Can you work these out from the model? Positions are in its coordinate system, mm. Face numbers are marked on the shaded views. A direction names the side the tool comes from. Round coordinates to 2 decimals unless told otherwise and drop trailing zeros. Order: outer loops, then holes, each group sorted by start corner. A loop starts at its lowest first (then second) coordinate and runs counter-clockwise, first axis right, second up.
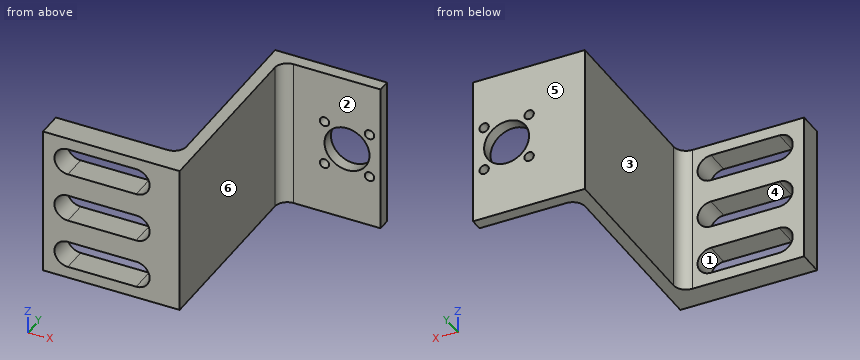
from build123d import *

# Parameters (mm, degrees)
BOSS_EXTRUDE1_DEPTH  = 19.05
FILLET1_R            = 3.175
SKETCH2_R            = 5.75
CUT_EXTRUDE1_DEPTH   = 4.175
M2_CLEARANCE_HOLE1_D = 2.4
CUT_EXTRUDE2_DEPTH   = 7.35
LPATTERN1_COUNT      = 2
LPATTERN1_PITCH      = 12.7
LPATTERN1_COL_COUNT  = 2
LPATTERN1_COL_PITCH  = 12.7


with BuildPart() as part:
    # Sketch1 → Boss-Extrude1 (new body, symmetric)
    with BuildSketch(Plane.XY):
        Polygon((-34.925, 0), (0, 0), (0, 50.2412), (25.4, 50.2412), (25.4, 53.4162), (-3.175, 53.4162), (-3.175, 6.35), (-34.925, 6.35), align=None)
    extrude(amount=BOSS_EXTRUDE1_DEPTH, both=True)

    # Fillet1
    fillet1_edges = [part.edges().sort_by_distance(p)[0] for p in [
        (-3.175, 6.35, 0),
        (0, 50.2412, 0),
    ]]
    fillet(fillet1_edges, radius=FILLET1_R)

    # Sketch2 → Cut-Extrude1 (cut, through all)
    with BuildSketch(Plane(origin=(16.8125, 50.2412, 0), x_dir=(1, 0, 0), z_dir=(0, -1, 0))):
        Circle(SKETCH2_R)
    extrude(amount=-CUT_EXTRUDE1_DEPTH, mode=Mode.SUBTRACT)

    # M2 Clearance Hole1 (through all)
    with Locations(Plane(origin=(16.8125, 50.2412, 0), x_dir=(-1, 0, 0), z_dir=(0, -1, 0))):
        with Locations((-5.75, -5.75), (-5.75, 5.75), (5.75, 5.75), (5.75, -5.75)):
            Hole(M2_CLEARANCE_HOLE1_D / 2)

    # Sketch5 → Cut-Extrude2 (cut, through all)
    with BuildSketch(Plane(origin=(0, 6.35, 0), x_dir=(1, 0, 0), z_dir=(0, 1, 0))):
        with BuildLine():
            Line((-28.575, 3.429), (-11.1125, 3.429))
            ThreePointArc((-11.1125, 3.429), (-7.6835, 0), (-11.1125, -3.429))
            Line((-11.1125, -3.429), (-28.575, -3.429))
            ThreePointArc((-28.575, -3.429), (-32.004, 0), (-28.575, 3.429))
        make_face()
    cut_extrude2 = extrude(amount=-CUT_EXTRUDE2_DEPTH, mode=Mode.SUBTRACT)

    # LPattern1: Cut-Extrude2 ×2
    with Locations(*[(0, 0, i * LPATTERN1_PITCH) for i in range(1, LPATTERN1_COUNT)]):
        add(cut_extrude2, mode=Mode.SUBTRACT)

    # LPattern1 col: Cut-Extrude2 ×2
    with Locations(*[(0, 0, -i * LPATTERN1_COL_PITCH) for i in range(1, LPATTERN1_COL_COUNT)]):
        add(cut_extrude2, mode=Mode.SUBTRACT)


solid = part.part
(1) I want a section at B-B, the plane z = 1. List the corners of the cut face in (x, y) for me (3 decimals).
(2) On a 3-axis mill with a long thin cutter (end or side, diameter ignored), from which of +Z, -Z, +X, -X, +Y, -Y can I reach the whole of each face in a straight line? I mean the marked faces 1, 2 and 3. Say none if no direction works.
(3) Please list where these lines run through material, in increasing order: probe 1 along X at (y, z) = (24, 8) (3 decimals); probe 2 along Y at (x, z) = (-8.5, 15); probe 3 along X at (y, z) = (51.5, 1) (3 decimals).
(4) If we mould it in two halves opening along X, with no side actions, what happens to the marked faces 4, 5 and 6? For each: pulls with the +X half, pulls with the -X half, needs draft (parallel to the pull), parting line crosses it, or undercut.
(5) I'm going to push flat-ended pins straight in: pin 1 Ø4 at (x, z) = (-6, 12.5) entering from +Y; pin 2 Ø12 at (y, z) = (25.5, 10.5) entering from +X; pin 3 Ø1.4 at (x, z) = (22.56, 5.75) entering from -Y; pin 4 Ø11 at (x, z) = (12.5, -7) entering from -Y. Where does each tip first touch, or does it pass through?
(6) I want a section at D-D, the plane x = 9. List the corners of the cut face in (y, z) for me.
(7) I want a section at C-C, the plane y = 16. List the corners of the cut face in (x, z) for me (3 decimals).
Ans:
1. outline: (-34.925, 0) - (-31.855, 0) - (-31.855, 6.35) - (-34.925, 6.35) - close; (-7.833, 0) - (0, 0) - (0, 47.066) arc R3.175 cw to (3.175, 50.241) - (11.15, 50.241) - (11.15, 53.416) - (-3.175, 53.416) - (-3.175, 9.525) arc R3.175 cw to (-6.35, 6.35) - (-7.833, 6.35) - close; (22.475, 50.241) - (25.4, 50.241) - (25.4, 53.416) - (22.475, 53.416) - close
2. face 1: +Y, -Y
2. face 2: +Z, -Z, +X, -Y
2. face 3: +Z, -Z, -X, +Y
3. probe 1: x = -3.175 to 0
3. probe 2: y = 0 to 6.35
3. probe 3: x = -3.175 to 11.15, 22.475 to 25.4
4. face 4: undercut
4. face 5: needs draft
4. face 6: pulls with the +X half
5. pin 1: stops at y = 7.39
5. pin 2: stops at x = 0
5. pin 3: passes through
5. pin 4: stops at y = 50.24
6. outline: (50.24, -19.05) - (53.42, -19.05) - (53.42, 19.05) - (50.24, 19.05) - close
7. outline: (-3.175, -19.05) - (0, -19.05) - (0, 19.05) - (-3.175, 19.05) - close
